Drawing for the job (mm, zero at the part's lowest x, y, z). Coordinates: 2 decimals unless noted, no trailing zeros. Write each loop counter-clockwise with the first axis right and the second up, starting at its lowest first coordinate (ties: lowest second). Pieces come first, ordered by that corner, then holes. Notation, with made-up numbers: M 87.5,82 L 108.5,82 A21 ccw 108.5,88 Z; hole C 44.5,33 d2. An arc over 180 degrees is marked long. Put each result on its own line as item: value. Start each with the question number.
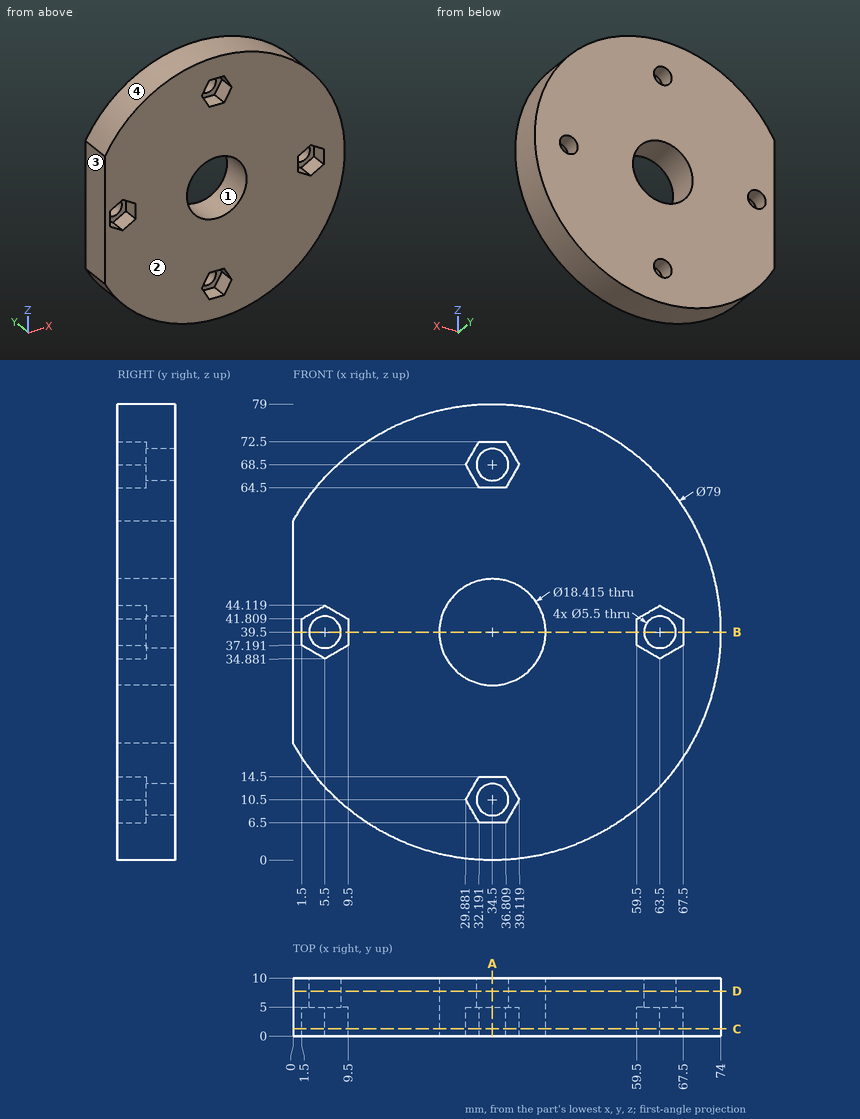
(1) Slice it at A-A, the plane x = 34.5. Write the cut outline in (y, z).
(2) Slice it at B-B, the plane z = 39.5. Write the cut outline in (x, y), then the cut area to 3 significant figures.
(3) Two-plate mould, pull along X, no slides. Class the marked faces 1, 2, 3 and 4: +X half, -X half, draft (parallel to the pull), parting line (faces both ways), or undercut.
(4) Slice it at D-D, the plane y = 7.75. State how many separate pieces and enclosed holes the cut face has, then the cut area to 3 significant figures.
(5) Drill centre lines: line 1 (Z direction, x = 34.5, y = 6.5); line 2 (Z direction, x = 36, y = 3.5) (1 decimal); line 3 (Z direction, x = 11, y = 2). Where is each one in solid material? Low to high. Write a range as [from, to].
(6) Slice it at C-C, the plane y = 1.25. Write the cut outline in (x, z) (1 decimal).
(7) Drop flat-ended pins along their axis: pin 1 (5 mm diameter, centred on x = 34, y = 3, fed in from +Z); pin 2 (5 mm diameter, centred on x = 42.5, y = 6, fed in from +Z) (1 decimal); pin 3 (6 mm diameter, centred on y = 3, z = 67.5, fed in from -X). Give the stop position or say it passes through.
Result set:
1. outline: M 0,0 L 10,0 L 10,7.75 L 5,7.75 L 5,6.5 L 0,6.5 Z; M 0,14.5 L 5,14.5 L 5,13.25 L 10,13.25 L 10,30.29 L 0,30.29 Z; M 0,48.71 L 10,48.71 L 10,65.75 L 5,65.75 L 5,64.5 L 0,64.5 Z; M 0,72.5 L 5,72.5 L 5,71.25 L 10,71.25 L 10,79 L 0,79 Z
2. outline: M 0,0 L 1.5,0 L 1.5,5 L 2.75,5 L 2.75,10 L 0,10 Z; M 8.25,5 L 9.5,5 L 9.5,0 L 25.29,0 L 25.29,10 L 8.25,10 Z; M 43.71,0 L 59.5,0 L 59.5,5 L 60.75,5 L 60.75,10 L 43.71,10 Z; M 66.25,5 L 67.5,5 L 67.5,0 L 74,0 L 74,10 L 66.25,10 Z
2. area: 421 mm^2
3. face 1: undercut
3. face 2: draft
3. face 3: -X half
3. face 4: parting line
4. separate pieces: 1
4. enclosed holes: 5
4. area: 4,410 mm^2
5. line 1: z = [0, 7.75], [13.25, 30.29], [48.71, 65.75], [71.25, 79]
5. line 2: z = [0, 6.5], [14.5, 30.4], [48.6, 64.5], [72.5, 79]
5. line 3: z = [7.75, 71.25]
6. outline: M 0,20.3 A39.5 ccw long 0,58.7 Z; hole M 1.5,37.2 L 5.5,34.9 L 9.5,37.2 L 9.5,41.8 L 5.5,44.1 L 1.5,41.8 Z; hole C 34.5,39.5 d18.4; hole M 29.9,10.5 L 32.2,6.5 L 36.8,6.5 L 39.1,10.5 L 36.8,14.5 L 32.2,14.5 Z; hole M 29.9,68.5 L 32.2,64.5 L 36.8,64.5 L 39.1,68.5 L 36.8,72.5 L 32.2,72.5 Z; hole M 59.5,37.2 L 63.5,34.9 L 67.5,37.2 L 67.5,41.8 L 63.5,44.1 L 59.5,41.8 Z
7. pin 1: stops at z = 79
7. pin 2: stops at z = 78.6
7. pin 3: stops at x = 3.92
